The model under review builds one solid part; all positions refer to its coordinate system, in mm. A direction names the side the tool comes from. Coordinates: 2 decimals unless noted, no trailing zeros. Order: outer loops, then holes, each group sorted by start corner. A loop starts at its lowest first (then second) coordinate and runs counter-clockwise, first axis right, second up. Notation, with made-up numbers: M -35,87.25 L 22,87.25 A28 ccw 22,108.25 Z; hole C -27,5 d6. An arc over 180 degrees is marked long. Write each question's results on one line, items separated by ' | '.
from build123d import *

# Parameters (mm, degrees)
F0_R     = 11
F1_DEPTH = 2.5
F2_SIZE2 = 1
F2_SIZE  = 1
F3_R     = 3.75
F4_DEPTH = 0.6
F5_R     = 1.9
F6_DEPTH = 6


with BuildPart() as f1:
    # F0 (on Top) → F1 (new body)
    with BuildSketch(Plane.XY):
        with Locations((0.425981, 0)):
            Circle(F0_R)
    extrude(amount=F1_DEPTH)

    # F2
    f2_edges = [f1.edges().sort_by_distance(p)[0] for p in [
        (-10.574019, 0, 0),
    ]]
    chamfer(f2_edges, length=F2_SIZE, length2=F2_SIZE2)

    # F3 (on face) → F4 (join)
    with BuildSketch(Plane.XY.offset(2.5)):
        Circle(F3_R)
    extrude(amount=F4_DEPTH)

    # F5 (on face) → F6 (join)
    with BuildSketch(Plane.XY.offset(3.1)):
        Circle(F5_R)
    extrude(amount=F6_DEPTH)


solid = f1.part
1) To check wall thickness, follow line 1 along Z through (x, y) = (-2, 5.25); line 2 along Y through (x, z) = (1, 8.25); line 3 along Y through (x, z) = (1.25, 5.5). State the ranges of each line that lie inside material, in increasing order.
Solutions:
line 1: 0 to 2.5 | line 2: -1.62 to 1.62 | line 3: -1.43 to 1.43
2) For pin 1 (1 mm diameter, centred on x = -1.5, z = 7, fed in from -Y); pin 2 (2 mm diameter, centred on x = 2.5, z = 8, fed in from -Y); pin 3 (8 mm diameter, centred on x = 5, y = 8.5, fed in from +Z), all flat-tipped, find the tip position at first contact; note any pin that passes through.
Solutions:
pin 1: y = -1.62 | pin 2: y = -1.17 | pin 3: z = 2.5
3) For faces 1 (the cylindrical face through (-1.9, 0.08, 6.06)), 2 (the flat face through (0, 0, 9.1)), list the 3-axis set-ups (+Z, -Z, +X, -X, +Y, -Y) from which the entire face can be reached by the end or side of a thin tool; tool diameter is ignored.
Solutions:
face 1: +Z | face 2: +Z, +X, -X, +Y, -Y
4) Take a section at B-B on z = 7.5. State the section outline as (x, y) points, plus the area to 3 significant figures.
Solutions:
outline: C 0,0 d3.8 | area: 11.3 mm2
5) Take a section at A-A on y = 0. State the section outline as (x, z) points, plus the area to 3 significant figures.
Solutions:
outline: M -10.57,1 L -9.57,0 L 10.43,0 L 11.43,1 L 11.43,2.5 L 3.75,2.5 L 3.75,3.1 L 1.9,3.1 L 1.9,9.1 L -1.9,9.1 L -1.9,3.1 L -3.75,3.1 L -3.75,2.5 L -10.57,2.5 Z | area: 81.3 mm2
